Can you work these out from the model? Positions are in its coordinate system, mm. Round coordinates to 2 decimals unless told otherwise and drop trailing zeros. Loops run counter-clockwise (first coordinate to the right, second up) from the corner with the lowest first, then second, coordinate; pieces in that order, holes last. Notation, with made-up numbers: M -7.75,31.25 L 29.25,31.25 A35 ccw 29.25,70.25 Z; hole C 28,35 d1. An arc over 180 degrees is marked long. Answer as CSV lines item,"result".
from build123d import *

# Parameters (mm, degrees)
F0_R     = 17.78
F0_W     = 50.8
F0_H     = 38.1
F0_R_2   = 7.62
F1_DEPTH = 10.414
F2_R     = 5.08


with BuildPart() as f1:
    # F0 (on Top) → F1 (new body)
    with BuildSketch(Plane.XY):
        with BuildLine():
            Line((-10.817469722, 14.821465837), (-61.617469722, 14.821465837))
            ThreePointArc((-61.617469722, 14.821465837), (-65.2095721705, 13.3335682854), (-66.697469722, 9.741465837))
            Line((-66.697469722, 9.741465837), (-66.697469722, -84.238534163))
            ThreePointArc((-66.697469722, -84.238534163), (-65.2095721705, -87.8306366114), (-61.617469722, -89.318534163))
            Line((-61.617469722, -89.318534163), (-10.817469722, -89.318534163))
            ThreePointArc((-10.817469722, -89.318534163), (-7.2253672736, -87.8306366114), (-5.737469722, -84.238534163))
            Line((-5.737469722, -84.238534163), (-5.737469722, 9.741465837))
            ThreePointArc((-5.737469722, 9.741465837), (-7.2253672736, 13.3335682854), (-10.817469722, 14.821465837))
        make_face()
        with Locations((-36.217469722, -58.838534163)):
            Circle(F0_R, mode=Mode.SUBTRACT)
        with Locations((-36.217469722, -10.578534163)):
            Rectangle(F0_W, F0_H, mode=Mode.SUBTRACT)
        with Locations((-36.217469722, -10.578534163)):
            Rectangle(F0_W, F0_H)
        with Locations((-36.217469722, -58.838534163)):
            Circle(F0_R)
        with Locations((-36.217469722, -58.838534163)):
            Circle(F0_R_2, mode=Mode.SUBTRACT)
        with Locations((-36.217469722, -58.838534163)):
            Circle(F0_R_2)
    extrude(amount=F1_DEPTH)

    # F2
    f2_edges = [f1.edges().sort_by_distance(p)[0] for p in [
        (-36.21747, -89.318534, 10.414),
        (-36.21747, 14.821466, 10.414),
    ]]
    fillet(f2_edges, radius=F2_R)


solid = f1.part
Item 1: If we section it at B-B on z = 9: Write out the boundary of the cut face in (x, y).
Output:
outline,"M -65.13,-84.24 A3.52 ccw -61.62,-87.76 L -10.82,-87.76 A3.52 ccw -7.3,-84.24 L -7.3,9.74 A3.52 ccw -10.82,13.26 L -61.62,13.26 A3.52 ccw -65.13,9.74 Z"
Item 2: Will this pin go through, and if not, where does the flat tip stop? pin 1 (10 mm diameter, centred on x = -36.5, y = -27.5, fed in from -Z).
Output:
pin 1,"stops at z = 0"
Item 3: If we section it at A-A on y = -73.5: Write out the boundary of the cut face in (x, z), then the cut area to 3 significant figures.
Output:
outline,"M -66.7,0 L -5.74,0 L -5.74,5.33 A5.08 ccw -10.82,10.41 L -61.62,10.41 A5.08 ccw -66.7,5.33 Z"
area,"624 mm2"
Item 4: If we section it at C-C on x = -63: Write out the boundary of the cut face in (y, z), then the cut area to 3 significant figures.
Output:
outline,"M -89.13,0 L 14.63,0 L 14.63,5.33 A4.89 ccw 9.74,10.22 L -84.24,10.22 A4.89 ccw -89.13,5.33 Z"
area,"1,050 mm2"
Item 5: If I drill on line 1 along Y through (x, z) = (-41, 5.75); line 2 along X through (y, z) = (-75, 8.75); line 3 along X through (y, z) = (-25, 9.5), over which ranges is the centre line in solid material (lowest first)? Write a range as from..to.
Output:
line 1,"y = -89.3..14.8"
line 2,"x = -65.38..-7.06"
line 3,"x = -64.52..-7.91"
